Input: part model. Units: mm. Frame: model coordinates. A direction names the side the tool comes from. Round coordinates to 2 decimals unless told otherwise and drop trailing zeros. Answer as a JSON object with one key per item and string values.
```python
from build123d import *

# Parameters (mm, degrees)
SKETCH1_R           = 2.5
BOSS_EXTRUDE1_DEPTH = 13.97
CUT_EXTRUDE1_REACH  = 108.146
SKETCH2_R           = 2.5
FILLET1_R           = 5
FILLET2_R           = 1
SKETCH3_R           = 2.5
CUT_EXTRUDE2_DEPTH  = 4


with BuildPart() as part:
    # Sketch1 → Boss-Extrude1 (new body)
    with BuildSketch(Plane(origin=(0, 0, 0), x_dir=(1, 0, 0), z_dir=(0, 1, 0))):
        Polygon((0, 7.071067812), (-7.071067812, 0), (62.778932188, -69.85), (81.2, -69.85), (81.2, -59.85), (66.921067812, -59.85), align=None)
        with Locations(Location((0, 0, 0), (0, 0, 270))):
            Circle(SKETCH1_R, mode=Mode.SUBTRACT)
    extrude(amount=BOSS_EXTRUDE1_DEPTH)

    # Sketch2 → Cut-Extrude1 (cut, up to next)
    with BuildSketch(Plane(origin=(0, 0, 59.85), x_dir=(-1, 0, 0), z_dir=(0, 0, -1)), mode=Mode.PRIVATE) as cut_extrude1_sk1:
        with Locations((-76.2, 6.35)):
            Circle(SKETCH2_R)
    cut_extrude1_tool1 = extrude(cut_extrude1_sk1.sketch, amount=-CUT_EXTRUDE1_REACH, mode=Mode.PRIVATE) & part.part
    add(cut_extrude1_tool1.solids().sort_by_distance((76.2, 6.35, 59.85))[0], mode=Mode.SUBTRACT)

    # Fillet1
    fillet1_edges = [part.edges().sort_by_distance(p)[0] for p in [
        (-7.071067812, 6.985, 0),
        (0, 6.985, -7.071067812),
        (81.2, 0, 64.85),
        (81.2, 13.97, 64.85),
        (62.778932188, 6.985, 69.85),
        (66.921067812, 6.985, 59.85),
    ]]
    fillet(fillet1_edges, radius=FILLET1_R - 0.0001)  # a hair under: the kernel refuses the full size

    # Fillet2
    fillet2_edges = [part.edges().sort_by_distance(p)[0] for p in [
        (28.889445383, 0, 35.960513195),
        (28.889445383, 13.97, 35.960513195),
        (70.525029289, 0, 69.85),
        (34.496047101, 0, 27.424979289),
        (72.596097101, 0, 59.85),
        (62.936579685, 0, 69.469405275),
        (0, 0, -5.000041421),
        (-5.000041421, 0, 0),
        (72.596097101, 13.97, 59.85),
        (34.496047101, 13.97, 27.424979289),
        (70.525029289, 13.97, 69.85),
        (62.936579685, 13.97, 69.469405275),
        (0, 13.97, -5.000041421),
        (-5.000041421, 13.97, 0),
        (81.2, 6.985, 59.85),
        (81.2, 6.985, 69.85),
        (79.735563195, 12.505563195, 59.85),
        (79.735563195, 1.464436805, 59.85),
        (79.735563195, 12.505563195, 69.85),
        (79.735563195, 1.464436805, 69.85),
        (67.078715309, 0, 59.469405275),
        (67.078715309, 13.97, 59.469405275),
    ]]
    fillet(fillet2_edges, radius=FILLET2_R)

    # Sketch3 → Cut-Extrude2 (cut)
    # profile 1 of 5: a face of its own
    with BuildSketch(Plane(origin=(0, 0, 59.85), x_dir=(-1, 0, 0), z_dir=(0, 0, -1))):
        with BuildLine():
            Line((-80.164228202, 4.466244658), (-78.725907428, 1.975))
            Line((-78.725907428, 1.975), (-73.674092572, 1.975))
            Line((-73.674092572, 1.975), (-71.148185145, 6.35))
            Line((-71.148185145, 6.35), (-73.674092572, 10.725))
            Line((-73.674092572, 10.725), (-78.725907428, 10.725))
            Line((-78.725907428, 10.725), (-80.2, 8.17179677))
            Line((-80.2, 8.17179677), (-80.2, 5))
            ThreePointArc((-80.2, 5), (-80.191047031, 4.732523652), (-80.164228202, 4.466244658))
        make_face()
        with Locations((-76.2, 6.35)):
            Circle(SKETCH3_R, mode=Mode.SUBTRACT)
    # profile 2 of 5: a face of its own
    with BuildSketch(Plane(origin=(0, 0, 59.85), x_dir=(-1, 0, 0), z_dir=(0, 0, -1))):
        with BuildLine():
            Line((-82.608963745, 1.975), (-78.817131063, 1.975))
            ThreePointArc((-78.817131063, 1.975), (-79.718543367, 3.097408985), (-80.164228202, 4.466244658))
            Line((-80.164228202, 4.466244658), (-81.251814855, 6.35))
            Line((-81.251814855, 6.35), (-80.2, 8.17179677))
            Line((-80.2, 8.17179677), (-80.2, 8.97))
            ThreePointArc((-80.2, 8.97), (-80.097290514, 9.870625701), (-79.794436674, 10.725))
            Line((-79.794436674, 10.725), (-82.608963745, 10.725))
            Line((-82.608963745, 10.725), (-82.608963745, 1.975))
        make_face()
    # profile 3 of 5: a face of its own
    with BuildSketch(Plane(origin=(0, 0, 59.85), x_dir=(-1, 0, 0), z_dir=(0, 0, -1))):
        with BuildLine():
            Line((-81.251814855, 6.35), (-80.164228202, 4.466244658))
            ThreePointArc((-80.164228202, 4.466244658), (-80.191047031, 4.732523652), (-80.2, 5))
            Line((-80.2, 5), (-80.2, 8.17179677))
            Line((-80.2, 8.17179677), (-81.251814855, 6.35))
        make_face()
    # profile 4 of 5: a face of its own
    with BuildSketch(Plane(origin=(0, 0, 59.85), x_dir=(-1, 0, 0), z_dir=(0, 0, -1))):
        with BuildLine():
            Line((-80.2, 8.97), (-80.2, 8.17179677))
            Line((-80.2, 8.17179677), (-78.725907428, 10.725))
            Line((-78.725907428, 10.725), (-79.794436674, 10.725))
            ThreePointArc((-79.794436674, 10.725), (-80.097290514, 9.870625701), (-80.2, 8.97))
        make_face()
    # profile 5 of 5: a face of its own
    with BuildSketch(Plane(origin=(0, 0, 59.85), x_dir=(-1, 0, 0), z_dir=(0, 0, -1))):
        with BuildLine():
            Line((-78.817131063, 1.975), (-78.725907428, 1.975))
            Line((-78.725907428, 1.975), (-80.164228202, 4.466244658))
            ThreePointArc((-80.164228202, 4.466244658), (-79.718543367, 3.097408985), (-78.817131063, 1.975))
        make_face()
    extrude(amount=-CUT_EXTRUDE2_DEPTH, mode=Mode.SUBTRACT)


solid = part.part
```
1) Contact query for flat-ended pins moving along their axis: P1, Ø7, axis at x = 75.5, y = 6, coming from the -Z side; P2, Ø2, axis at x = 54, y = 12, coming from the +Z side; P3, Ø4, axis at y = 10.5, z = 31.5, coming from the +X side. Output: stop coordinate, or through.
Output:
{"P1": "stops at z = 63.85", "P2": "stops at z = 62.07", "P3": "stops at x = 40.57"}
2) Draft query along Y for faces 1 (the face through (34.72, 13.68, 28.07)), 2 (the face through (81.2, 7, 66)), 3 (the face through (78.5, 8.4, 63.85)), 4 (the face through (29.556, 0.285, 36.202)). Return one class per face: +Y half, -Y half, draft (parallel to the pull), parting line (faces both ways), or undercut.
Output:
{"face 1": "+Y half", "face 2": "draft", "face 3": "undercut", "face 4": "-Y half"}
3) Ray query, probe 1 along Y at (x, z) = (76.2, 66.5); probe 2 along X at (y, z) = (12, -0.5); probe 3 along X at (y, z) = (12.75, 48.5). Return the intervals inside material, ascending.
Output:
{"probe 1": "y = 0 to 3.85, 8.85 to 13.97", "probe 2": "x = -4.97 to -2.45, 2.45 to 6.57", "probe 3": "x = 41.43 to 55.57"}
4) Section A-A, the plane y = 7.5. Count the separate pieces of the cut face and the enclosed holes in it, plus the area to 3 significant figures.
Output:
{"separate pieces": "2", "enclosed holes": "1", "area": "1,040 mm^2"}
5) Reachability of faces 5 (the face through (77, 1.975, 62)), 6 (the face through (71, 7, 59.85)), 7 (the face through (-2.44, 6.89, -0.54)) from +Z, -Z, +X, -X, +Y, -Y: full face, straight path, thin tool, end or side. Return the list, or none.
Output:
{"face 5": "-Z, +X", "face 6": "-Z, +X, +Y, -Y", "face 7": "+Y, -Y"}
